Source: CAD feature listing. Evaluate the final solid. Frame: model axes, mm. A direction names the side the tool comes from. Give positions to 0.01 mm unless a question says otherwise; leave off trailing zeros. Loops run counter-clockwise (first coordinate to the right, second up) from the corner with the lowest first, then second, coordinate; pieces in that order, holes last. Notation, with made-up numbers: M 83.25,30 L 91.25,30 A14 ccw 91.25,56 Z; hole C -19.75,-11 d11. An arc over 180 degrees is marked long. Answer in a Markdown table with one row per item.
```python
from build123d import *

# Parameters (mm, degrees)
SKETCH1_R           = 21.25
BOSS_EXTRUDE1_DEPTH = 150
SKETCH2_R           = 45
BOSS_EXTRUDE2_DEPTH = 5
SHELL1_T            = -1


with BuildPart() as part:
    # Sketch1 → Boss-Extrude1 (new body)
    with BuildSketch(Plane.XY):
        Circle(SKETCH1_R)
    extrude(amount=BOSS_EXTRUDE1_DEPTH)

    # Sketch2 → Boss-Extrude2 (add)
    with BuildSketch(Plane.XY.offset(150)):
        Circle(SKETCH2_R)
    extrude(amount=BOSS_EXTRUDE2_DEPTH)

    # Sketch4 → Revolve1 (revolve)
    with BuildSketch(Plane(origin=(0, 0, 0), x_dir=(0, 0, -1), z_dir=(1, 0, 0)), mode=Mode.PRIVATE) as revolve1_sk:
        Polygon((0, 21.25), (6.8, 5.35), (40.8, 3.25), (40.8, 0), (0, 0), align=None)
    revolve(revolve1_sk.sketch.rotate(Axis((0, 0, 0), (0, 0, -1)), 90), axis=Axis((0, 0, 0), (0, 0, -1)))

    # Shell1
    shell1_openings = [part.faces().sort_by_distance(p)[0] for p in [
        (0, 0, 155),
    ]]
    offset(amount=SHELL1_T, openings=shell1_openings, kind=Kind.INTERSECTION)


solid = part.part
```
Q1. Section query C-C (z = 90.5). Output: boundary loops of the cut face in (x, y), plus the area to 3 significant figures.
Values follow:
| item | result |
|---|---|
| outline | C 0,0 d42.5; hole C 0,0 d40.5 |
| area | 130 mm^2 |
Q2. Mould query, pull axis Y, two halves, no side actions, for faces 4 (the flat face through (0, 0, -40.8)), 5 (the conical face through (-4.86, 3.73, -6.47)), 6 (the flat face through (0, 0, -39.8)). Classes: +Y half, -Y half, draft (parallel to the pull), parting line (faces both ways), or undercut.
Values follow:
| item | result |
|---|---|
| face 4 | draft |
| face 5 | parting line |
| face 6 | undercut |
Q3. Ray query, probe 1 along Y at (x, z) = (0, 152); probe 2 along Y at (x, z) = (0, 52); probe 3 along Z at (x, y) = (-10.5, 25). Return the intervals inside material, ascending. Write a range as from..to.
Values follow:
| item | result |
|---|---|
| probe 1 | -45..-44, 44..45 |
| probe 2 | -21.25..-20.25, 20.25..21.25 |
| probe 3 | 150..151 |
Q4. Contact query for flat-ended pins moving along their axis: pin 1 Ø10 at (x, y) = (-19.5, 8.5) entering from -Z; pin 2 Ø4 at (y, z) = (-17.5, 54.5) entering from -X; pin 3 Ø8 at (x, y) = (17, 27.5) entering from +Z. Output: stop coordinate, or through.
Values follow:
| item | result |
|---|---|
| pin 1 | z = -2.13 |
| pin 2 | x = -14.54 |
| pin 3 | z = 151 |
Q5. Section query A-A (x = 0). Output: boundary loops of the cut face in (y, z), plus the area to 3 significant figures.
Values follow:
| item | result |
|---|---|
| outline | M -45,150 L -21.25,150 L -21.25,0 L -5.35,-6.8 L -3.25,-40.8 L 3.25,-40.8 L 5.35,-6.8 L 21.25,0 L 21.25,150 L 45,150 L 45,155 L 44,155 L 44,151 L 20.25,151 L 20.25,0.66 L 4.39,-6.12 L 2.31,-39.8 L -2.31,-39.8 L -4.39,-6.12 L -20.25,0.66 L -20.25,151 L -44,151 L -44,155 L -45,155 Z |
| area | 465 mm^2 |
Q6. Reachability of faces 1 (the cylindrical face through (-16.863, -12.93, 73.95)), 2 (the cylindrical face through (20.765, -39.923, 152.465)), 3 (the flat face through (9, -19, 151)) from +Z, -Z, +X, -X, +Y, -Y: full face, straight path, thin tool, end or side. Return the list, or none.
Values follow:
| item | result |
|---|---|
| face 1 | -Z |
| face 2 | +Z, -Z |
| face 3 | +Z |
Q7. Section query D-D (x = 24.5). Output: boundary loops of the cut face in (y, z), plus the area to 3 significant figures.
Values follow:
| item | result |
|---|---|
| outline | M -37.75,150 L 37.75,150 L 37.75,155 L 36.55,155 L 36.55,151 L -36.55,151 L -36.55,155 L -37.75,155 Z |
| area | 85.1 mm^2 |
